CAD build for the part. Positions are in the model's coordinates, mm. Face numbers are marked on the shaded views. Give positions to 0.01 mm unless a question says otherwise; leave off trailing zeros. Write each loop counter-clockwise with the first axis right and the second up, starting at its lowest first coordinate (ties: lowest second). Pieces come first, ordered by that corner, then holes. Notation, with made-up numbers: (23, 60.5) - (75, 60.5) arc R23 cw to (75, 87.5) - close; hole circle Ø4 at (-18.5, 66.5). An arc over 180 degrees is marked (long way). Put each result on its own line as item: value. Start each with the question number.
1. Mould opens along X. For the marked faces 1 and 2 say: +X half, -X half, draft (parallel to the pull), parting line (faces both ways), or undercut.
2. Cut at D-D on z = -22. List the corners of the cut face in (x, y), and give its area (3 significant figures).
3. Wall check: line 1 (X direction, y = 7.85, z = -37.7); line 2 (X direction, y = 5.1, z = -37.7); line 3 (Y direction, x = 5, z = -10). Give the ranges that are in metal, low to high.
4. Cut at C-C on z = -37.7. List the corners of the cut face in (x, y), and give its area (3 significant figures).
5. Drop flat-ended pins along their axis: pin 1 (5 mm diameter, centred on x = 38.5, y = 1, fed in from +Z); pin 2 (1.5 mm diameter, centred on x = 37.5, z = -37.5, fed in from +Y). Give the stop position or say it passes through.
6. Cut at B-B on x = 37.7. List the corners of the cut face in (y, z), and give its area (3 significant figures).
7. Cut at A-A on y = 8.25. List the corners of the cut face in (x, z), and give its area (3 significant figures).
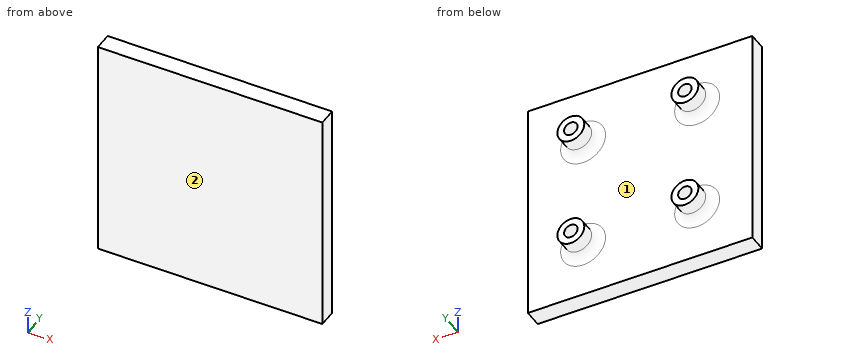
from build123d import *

# Parameters (mm, degrees)
SKETCH2_W                 = 50
SKETCH2_H                 = 50
BOSS_EXTRUDE1_DEPTH       = 4
SKETCH3_R                 = 1.5
CUT_EXTRUDE1_DEPTH        = 4
BOSS_EXTRUDE2_START       = 5
SKETCH4_R                 = 3
SKETCH4_R_2               = 1.5
BOSS_EXTRUDE2_DEPTH       = 5
MIRROR2_START             = 5
MIRROR2_COPY_1_SKETCH_R   = 3
MIRROR2_COPY_1_SKETCH_R_2 = 1.5
MIRROR2_COPY_1_DEPTH      = 5
FILLET1_R                 = 2
SKETCH6_W                 = 50
SKETCH6_H                 = 50
BOSS_EXTRUDE3_DEPTH       = 4


with BuildPart() as part:
    # Sketch2 → Boss-Extrude1 (new body)
    with BuildSketch(Plane(origin=(0, 0, 0), x_dir=(1, 0, 0), z_dir=(0, 1, 0))):
        with Locations((25, 25)):
            Rectangle(SKETCH2_W, SKETCH2_H)
    extrude(amount=BOSS_EXTRUDE1_DEPTH)

    # Sketch3 → Cut-Extrude1 (cut)
    with BuildSketch(Plane(origin=(0, 4, 0), x_dir=(1, 0, 0), z_dir=(0, 1, 0))):
        with Locations(Location((12.3, 37.7, 0), (0, 0, 270))):
            Circle(SKETCH3_R)
        with Locations(Location((12.3, 12.3, 0), (0, 0, 270))):
            Circle(SKETCH3_R)
        with Locations(Location((37.7, 37.7, 0), (0, 0, 270))):
            Circle(SKETCH3_R)
        with Locations(Location((37.7, 12.3, 0), (0, 0, 270))):
            Circle(SKETCH3_R)
    extrude(amount=-CUT_EXTRUDE1_DEPTH, mode=Mode.SUBTRACT)

    # Sketch4 → Boss-Extrude2 (add)
    with BuildSketch(Plane(origin=(0, 4, 0), x_dir=(1, 0, 0), z_dir=(0, 1, 0)).offset(BOSS_EXTRUDE2_START)):
        with Locations(Location((12.3, 37.7, 0), (0, 0, 90))):
            Circle(SKETCH4_R)
        with Locations(Location((12.3, 37.7, 0), (0, 0, 270))):
            Circle(SKETCH4_R_2, mode=Mode.SUBTRACT)
    boss_extrude2 = extrude(amount=-BOSS_EXTRUDE2_DEPTH)

    # Mirror1: Boss-Extrude2 across plane
    add(boss_extrude2.mirror(Plane.XY.offset(-25)))

    # Mirror2: Boss-Extrude2 across plane
    add(boss_extrude2.mirror(Plane.ZY.offset(-25)))

    # Mirror2 copy 1 sketch → Mirror2 copy 1 (add)
    with BuildSketch(Plane(origin=(50, 4, -50), x_dir=(-1, 0, 0), z_dir=(0, 1, 0)).offset(MIRROR2_START)):
        with Locations(Location((12.3, 37.7, 0), (0, 0, 90))):
            Circle(MIRROR2_COPY_1_SKETCH_R)
        with Locations(Location((12.3, 37.7, 0), (0, 0, 270))):
            Circle(MIRROR2_COPY_1_SKETCH_R_2, mode=Mode.SUBTRACT)
    extrude(amount=-MIRROR2_COPY_1_DEPTH)

    # Fillet1
    fillet1_edges = [part.edges().sort_by_distance(p)[0] for p in [
        (12.3, 4, -34.7),
        (12.3, 4, -15.3),
        (37.7, 4, -15.3),
        (37.7, 4, -34.7),
    ]]
    fillet(fillet1_edges, radius=FILLET1_R)

    # Sketch6 → Boss-Extrude3 (add)
    with BuildSketch(Plane.XZ):
        with Locations((25, -25)):
            Rectangle(SKETCH6_W, SKETCH6_H)
    extrude(amount=-BOSS_EXTRUDE3_DEPTH)


solid = part.part
Report:
1. face 1: undercut
1. face 2: draft
2. outline: (0, 0) - (50, 0) - (50, 4) - (0, 4) - close
2. area: 200 mm²
3. line 1: x = 9.3 to 10.8, 13.8 to 15.3, 34.7 to 36.2, 39.2 to 40.7
3. line 2: x = 9.09 to 10.8, 13.8 to 15.51, 34.49 to 36.2, 39.2 to 40.91
3. line 3: y = 0 to 4
4. outline: (0, 0) - (50, 0) - (50, 4) - (42.7, 4) arc R2 cw to (40.7, 6) - (40.7, 9) - (39.2, 9) - (39.2, 4) - (36.2, 4) - (36.2, 9) - (34.7, 9) - (34.7, 6) arc R2 cw to (32.7, 4) - (17.3, 4) arc R2 cw to (15.3, 6) - (15.3, 9) - (13.8, 9) - (13.8, 4) - (10.8, 4) - (10.8, 9) - (9.3, 9) - (9.3, 6) arc R2 cw to (7.3, 4) - (0, 4) - close
4. area: 233 mm²
5. pin 1: stops at z = 0
5. pin 2: stops at y = 4
6. outline: (0, -50) - (4, -50) - (4, -42.7) arc R2 cw to (6, -40.7) - (9, -40.7) - (9, -39.2) - (4, -39.2) - (4, -36.2) - (9, -36.2) - (9, -34.7) - (6, -34.7) arc R2 cw to (4, -32.7) - (4, -17.3) arc R2 cw to (6, -15.3) - (9, -15.3) - (9, -13.8) - (4, -13.8) - (4, -10.8) - (9, -10.8) - (9, -9.3) - (6, -9.3) arc R2 cw to (4, -7.3) - (4, 0) - (0, 0) - close
6. area: 233 mm²
7. outline: circle Ø6 at (12.3, -37.7); circle Ø6 at (12.3, -12.3); circle Ø6 at (37.7, -37.7); circle Ø6 at (37.7, -12.3); hole circle Ø3 at (12.3, -37.7); hole circle Ø3 at (12.3, -12.3); hole circle Ø3 at (37.7, -37.7); hole circle Ø3 at (37.7, -12.3)
7. area: 84.8 mm²
